Could you check a few things on this model? Use its own coordinates, in mm. Round coordinates to 2 decimals unless told otherwise and drop trailing zeros. Use one line per item in the form item = value.
```python
from build123d import *

# Parameters (mm, degrees)
BOSS_EXTRUDE2_DEPTH = 600


with BuildPart() as part:
    # Sketch1 → Boss-Extrude2 (new body)
    with BuildSketch(Plane(origin=(0, 0, 0), x_dir=(1, 0, 0), z_dir=(0, 1, 0))):
        with BuildLine():
            Line((23.9, 20), (23.9, 17.160660172))
            Line((23.9, 17.160660172), (26.560660172, 14.5))
            Line((26.560660172, 14.5), (28.2, 14.5))
            Line((28.2, 14.5), (28.2, 16.9))
            Line((28.2, 16.9), (29.5, 16.9))
            Line((29.5, 16.9), (29.5, 16.4))
            Line((29.5, 16.4), (30, 16.4))
            Line((30, 16.4), (30, 10.75))
            Line((30, 10.75), (30, 9.25))
            Line((30, 9.25), (30, 3.6))
            Line((30, 3.6), (29.5, 3.6))
            Line((29.5, 3.6), (29.5, 3.1))
            Line((29.5, 3.1), (28.2, 3.1))
            Line((28.2, 3.1), (28.2, 5.5))
            Line((28.2, 5.5), (26.560660172, 5.5))
            Line((26.560660172, 5.5), (23.9, 2.839339828))
            Line((23.9, 2.839339828), (23.9, 0))
            Line((23.9, 0), (23.9, -2.839339828))
            Line((23.9, -2.839339828), (26.560660172, -5.5))
            Line((26.560660172, -5.5), (28.2, -5.5))
            Line((28.2, -5.5), (28.2, -3.1))
            Line((28.2, -3.1), (29.5, -3.1))
            Line((29.5, -3.1), (29.5, -3.6))
            Line((29.5, -3.6), (30, -3.6))
            Line((30, -3.6), (30, -9.25))
            ThreePointArc((30, -9.25), (29.780330086, -9.780330086), (29.25, -10))
            Line((29.25, -10), (25.5, -10))
            Line((25.5, -10), (23.6, -10))
            Line((23.6, -10), (23.6, -9.5))
            Line((23.6, -9.5), (23.1, -9.5))
            Line((23.1, -9.5), (23.1, -8.2))
            Line((23.1, -8.2), (25.5, -8.2))
            Line((25.5, -8.2), (25.5, -6.560660172))
            Line((25.5, -6.560660172), (22.839339828, -3.9))
            Line((22.839339828, -3.9), (17.160660172, -3.9))
            Line((17.160660172, -3.9), (14.5, -6.560660172))
            Line((14.5, -6.560660172), (14.5, -8.2))
            Line((14.5, -8.2), (16.9, -8.2))
            Line((16.9, -8.2), (16.9, -9.5))
            Line((16.9, -9.5), (16.4, -9.5))
            Line((16.4, -9.5), (16.4, -10))
            Line((16.4, -10), (14.5, -10))
            Line((14.5, -10), (10.75, -10))
            ThreePointArc((10.75, -10), (10.219669914, -9.780330086), (10, -9.25))
            Line((10, -9.25), (10, -3.6))
            Line((10, -3.6), (10.5, -3.6))
            Line((10.5, -3.6), (10.5, -3.1))
            Line((10.5, -3.1), (11.8, -3.1))
            Line((11.8, -3.1), (11.8, -5.5))
            Line((11.8, -5.5), (13.439339828, -5.5))
            Line((13.439339828, -5.5), (16.1, -2.839339828))
            Line((16.1, -2.839339828), (16.1, 0))
            Line((16.1, 0), (16.1, 2.839339828))
            Line((16.1, 2.839339828), (13.439339828, 5.5))
            Line((13.439339828, 5.5), (11.8, 5.5))
            Line((11.8, 5.5), (11.8, 3.1))
            Line((11.8, 3.1), (10.5, 3.1))
            Line((10.5, 3.1), (10.5, 3.6))
            Line((10.5, 3.6), (10, 3.6))
            Line((10, 3.6), (10, 9.25))
            Line((10, 9.25), (10, 10.75))
            Line((10, 10.75), (10, 16.4))
            Line((10, 16.4), (10.5, 16.4))
            Line((10.5, 16.4), (10.5, 16.9))
            Line((10.5, 16.9), (11.8, 16.9))
            Line((11.8, 16.9), (11.8, 14.5))
            Line((11.8, 14.5), (13.439339828, 14.5))
            Line((13.439339828, 14.5), (16.1, 17.160660172))
            Line((16.1, 17.160660172), (16.1, 20))
            Line((16.1, 20), (16.1, 22.839339828))
            Line((16.1, 22.839339828), (13.439339828, 25.5))
            Line((13.439339828, 25.5), (11.8, 25.5))
            Line((11.8, 25.5), (11.8, 23.1))
            Line((11.8, 23.1), (10.5, 23.1))
            Line((10.5, 23.1), (10.5, 23.6))
            Line((10.5, 23.6), (10, 23.6))
            Line((10, 23.6), (10, 29.25))
            ThreePointArc((10, 29.25), (10.219669914, 29.780330086), (10.75, 30))
            Line((10.75, 30), (14.5, 30))
            Line((14.5, 30), (16.4, 30))
            Line((16.4, 30), (16.4, 29.5))
            Line((16.4, 29.5), (16.9, 29.5))
            Line((16.9, 29.5), (16.9, 28.2))
            Line((16.9, 28.2), (14.5, 28.2))
            Line((14.5, 28.2), (14.5, 26.560660172))
            Line((14.5, 26.560660172), (17.160660172, 23.9))
            Line((17.160660172, 23.9), (22.839339828, 23.9))
            Line((22.839339828, 23.9), (25.5, 26.560660172))
            Line((25.5, 26.560660172), (25.5, 28.2))
            Line((25.5, 28.2), (23.1, 28.2))
            Line((23.1, 28.2), (23.1, 29.5))
            Line((23.1, 29.5), (23.6, 29.5))
            Line((23.6, 29.5), (23.6, 30))
            Line((23.6, 30), (25.5, 30))
            Line((25.5, 30), (29.25, 30))
            ThreePointArc((29.25, 30), (29.780330086, 29.780330086), (30, 29.25))
            Line((30, 29.25), (30, 23.6))
            Line((30, 23.6), (29.5, 23.6))
            Line((29.5, 23.6), (29.5, 23.1))
            Line((29.5, 23.1), (28.2, 23.1))
            Line((28.2, 23.1), (28.2, 25.5))
            Line((28.2, 25.5), (26.560660172, 25.5))
            Line((26.560660172, 25.5), (23.9, 22.839339828))
            Line((23.9, 22.839339828), (23.9, 20))
        make_face()
        Polygon((17.160660172, 16.1), (13.760660172, 12.7), (11.8, 12.7), (11.8, 7.3), (13.760660172, 7.3), (17.160660172, 3.9), (22.839339828, 3.9), (26.239339828, 7.3), (28.2, 7.3), (28.2, 12.7), (26.239339828, 12.7), (22.839339828, 16.1), align=None, mode=Mode.SUBTRACT)
        with BuildLine():
            ThreePointArc((22.5, 20), (20, 17.5), (17.5, 20))
            ThreePointArc((17.5, 20), (20, 22.5), (22.5, 20))
        make_face(mode=Mode.SUBTRACT)
        with BuildLine():
            ThreePointArc((22.5, 0), (20, -2.5), (17.5, 0))
            ThreePointArc((17.5, 0), (20, 2.5), (22.5, 0))
        make_face(mode=Mode.SUBTRACT)
    extrude(amount=BOSS_EXTRUDE2_DEPTH)


solid = part.part
```
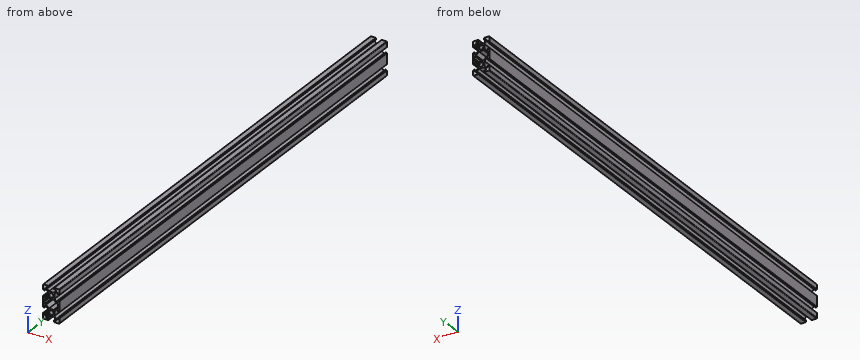
1. For P1, Ø8, axis at y = 310.5, z = -20.5, coming from the +X side; P2, Ø2, axis at x = 21.5, y = 379.5, coming from the -Z side; P3, Ø4, axis at x = 16.5, z = -8.5, coming from the -Y side, each with a flat end and sliding along its axis, tell me the tip position at first contact or that it passes through.
Solution:
P1 = 30
P2 = -23.9
P3 = through
2. Please list where these lines run through material, in increasing order: line 1 along Z through (x, y) = (27.75, 183.5); line 2 along Z through (x, y) = (20, 417.5); line 3 along X through (y, z) = (249.5, -20).
Solution:
line_1 = -30 to -25.5, -14.5 to -12.7, -7.3 to -5.5, 5.5 to 10
line_2 = -23.9 to -22.5, -17.5 to -16.1, -3.9 to -2.5, 2.5 to 3.9
line_3 = 16.1 to 17.5, 22.5 to 23.9
3. If we section it at A-A, the plane y = 99: Count the separate pieces of the cut face and the enclosed holes in it, plus the area to 3 significant figures.
Solution:
separate_pieces = 1
enclosed_holes = 3
area = 299 mm^2
